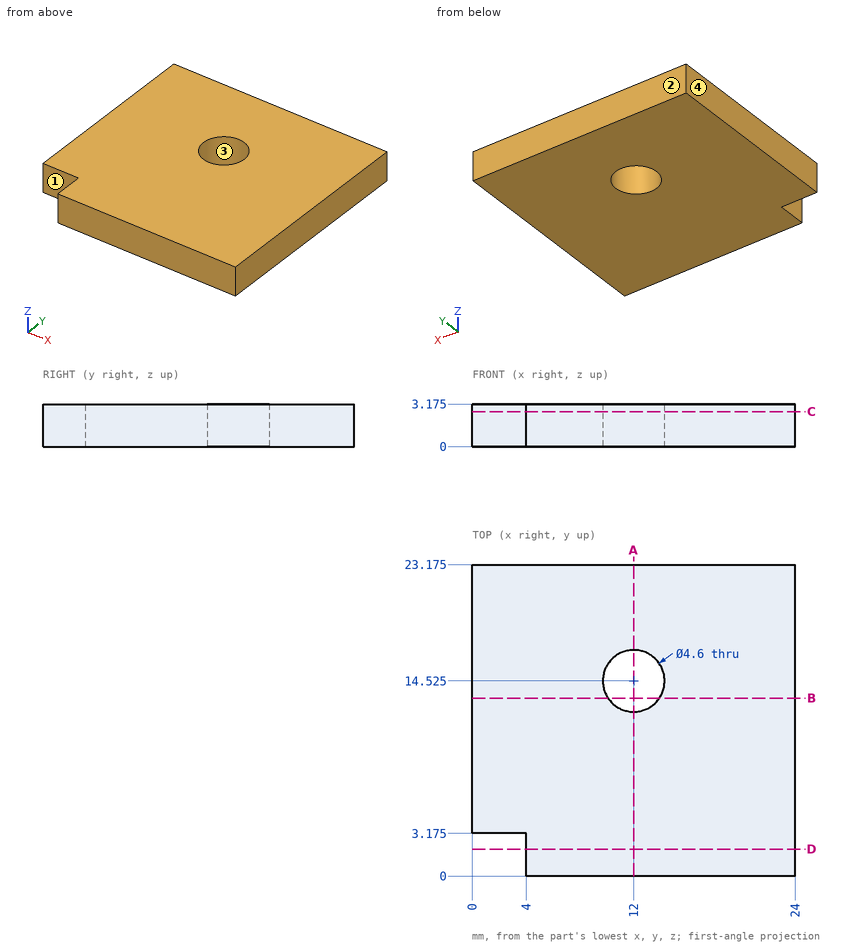
Job drawing, mm, ordinate dimensions from the low corner. One solid piece. Coordinates: 2 decimals unless noted, no trailing zeros. Order: outer loops, then holes, each group sorted by start corner. A loop starts at its lowest first (then second) coordinate and runs counter-clockwise, first axis right, second up. Notation, with made-up numbers: M 51,78 L 110,78 A18 ccw 110,100 Z; hole C -21.5,34 d9. An arc over 180 degrees is marked long. Return JSON: item names as keys, results as strings.
1. Saw through at C-C (z = 2.6). Give the cut face in (x, y) (3 decimals).
Ans:
{"outline": "M 0,3.175 L 4,3.175 L 4,0 L 24,0 L 24,23.175 L 0,23.175 Z; hole C 12,14.525 d4.6"}
2. Drill centre lines: probe 1 along Y at (x, z) = (12, 1.2) (3 decimals); probe 2 along X at (y, z) = (13.5, 1.5); probe 3 along Y at (x, z) = (1, 1.25) (3 decimals). Where is each one in solid material? Low to high.
Ans:
{"probe 1": "0 to 12.225, 16.825 to 23.175", "probe 2": "0 to 9.94, 14.06 to 24", "probe 3": "3.175 to 23.175"}
3. Flat gauge pins, fed straight in: pin 1 (1.6 mm diameter, centred on x = 2.5, z = 1.5, fed in from -Y) (3 decimals); pin 2 (6 mm diameter, centred on x = 12, y = 14.525, fed in from +Z) (3 decimals); pin 3 (1 mm diameter, centred on y = 1.5, z = 1.5, fed in from -X). Where does each tip first touch, or does it go through?
Ans:
{"pin 1": "y = 3.175", "pin 2": "z = 3.175", "pin 3": "x = 4"}
4. Saw through at D-D (y = 2). Give the cut face in (x, z) (3 decimals).
Ans:
{"outline": "M 4,0 L 24,0 L 24,3.175 L 4,3.175 Z"}
5. Pull direction Y, two halves, no side cores. Call the marked faces 1, 2, 3 and 4: +Y half, -Y half, draft (parallel to the pull), parting line (faces both ways), or undercut.
Ans:
{"face 1": "-Y half", "face 2": "+Y half", "face 3": "undercut", "face 4": "draft"}
6. Saw through at B-B (y = 13.25). Give the cut face in (x, z) (3 decimals), and give its area (3 significant figures).
Ans:
{"outline": "M 0,0 L 10.086,0 L 10.086,3.175 L 0,3.175 Z; M 13.914,0 L 24,0 L 24,3.175 L 13.914,3.175 Z", "area": "64.0 mm^2"}
7. Saw through at A-A (x = 12). Give the cut face in (y, z) (3 decimals), and give its area (3 significant figures).
Ans:
{"outline": "M 0,0 L 12.225,0 L 12.225,3.175 L 0,3.175 Z; M 16.825,0 L 23.175,0 L 23.175,3.175 L 16.825,3.175 Z", "area": "59.0 mm^2"}
